Here's how the part is built. I have some questions about the finished solid (model axes, mm). Face numbers are marked on the shaded views. Give positions to 0.01 mm unless a question says otherwise; leave off trailing zeros. Loops run counter-clockwise (first coordinate to the right, second up) from the corner with the lowest first, then second, coordinate; pieces in that order, holes last. Notation, with made-up numbers: (-14, 63) - (-5, 63) arc R20 ccw to (-5, 93) - close; hole circle Ø10 at (64, 58). An arc over 180 degrees is marked (long way). Use one line per item in the form item = value.
Autodesk Inventor part; units mm, degrees
ref_plane "YZ Plane" through (0, 0, 0) normal (1, 0, 0) x (0, 1, 0)
ref_plane "XZ Plane" through (0, 0, 0) normal (0, 1, 0) x (-1, 0, 0)
ref_plane "XY Plane" through (0, 0, 0) normal (0, 0, 1) x (1, 0, 0)
sketch "Sketch1" plane through (0, 0, 0) normal (0, 0, 1) x (1, 0, 0)
  line L0 (0, 31.75) -> (12.7, 31.75)
  line L1 (12.7, 31.75) -> (12.7, -31.75)
  line L2 (12.7, -31.75) -> (0, -31.75)
  line L3 (0, -31.75) -> (0, 31.75)
  point P0 (0, 0)
  point P1 (0, 0)
  dimension "d0" = 25.4
  dimension "d1" = 63.5
revolve "Revolution1" add sketch "Sketch1" angle 360 about axis through (0, -31.75, 0) along (0, 1, 0)
sketch "Sketch2" plane through (0, 0, 0) normal (0, 0, 1) x (1, 0, 0)
  line L0 (0, -35.56) -> (0, 35.56)
  line L1 (0, 25.4) -> (60.325, 25.4)
  line L2 (60.325, 25.4) -> (60.325, -25.4)
  line L3 (60.325, -25.4) -> (0, -25.4)
  line L4 (0, -25.4) -> (0, 25.4)
  circle A0 centre (60.325, 0) radius 25.4
  point P0 (0, 0)
  dimension "d3" = 60.325
  dimension "d4" = 50.8
extrude "Extrusion1" add sketch "Sketch2" along normal mid plane 25.4
sketch "Sketch3" plane through (0, 31.75, 0) normal (0, 1, 0) x (1, 0, 0)
  circle A0 centre (0, 0) radius 12.7
  circle A1 centre (0, 0) radius 7.9375
  dimension "d7" = 15.875
extrude "Extrusion2" cut sketch "Sketch3" against normal through all contours A1
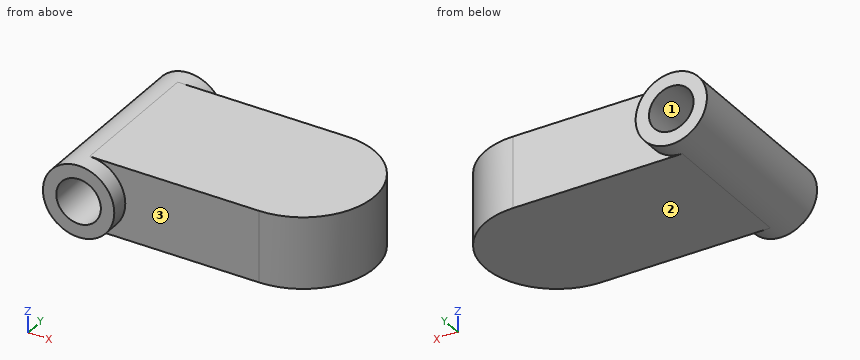
(1) If we section it at B-B (y = 0): List the corners of the cut face in (x, z) for me (1 decimal), plus the area to 3 significant figures.
Geometry says:
outline = (0, -12.7) - (85.7, -12.7) - (85.7, 12.7) - (0, 12.7) arc R12.7 ccw to start; hole circle Ø15.9 at (0, 0)
area = 2,230 mm²
(2) If we section it at D-D (x = 57.5): List the corners of the cut face in (y, z) for me.
Geometry says:
outline = (-25.4, -12.7) - (25.4, -12.7) - (25.4, 12.7) - (-25.4, 12.7) - close
(3) If I drill on probe 1 along Z at (x, y) = (0, -17); probe 2 along X at (y, z) = (12.5, -5); probe 3 along X at (y, z) = (14, 0), over which ranges is the centre line in solid material (lowest first)?
Geometry says:
probe_1 = -12.7 to -7.94, 7.94 to 12.7
probe_2 = -11.67 to -6.16, 6.16 to 82.44
probe_3 = -12.7 to -7.94, 7.94 to 81.52
(4) If we section it at C-C (x = -3): List the corners of the cut face in (y, z) for me.
Geometry says:
outline = (-31.75, -12.34) - (31.75, -12.34) - (31.75, -7.35) - (-31.75, -7.35) - close; (-31.75, 7.35) - (31.75, 7.35) - (31.75, 12.34) - (-31.75, 12.34) - close
(5) For P1, Ø12.5, axis at x = 39, z = -3, coming from the +Y side; P2, Ø5, axis at y = -5, z = 9, coming from the +X side; P3, Ø2, axis at y = -11.5, z = 5.5, coming from the -X side, each with a flat end and sliding along its axis, tell me the tip position at first contact or that it passes through.
Geometry says:
P1 = 25.4
P2 = 85.6
P3 = -11.88
(6) Thinking about a two-plate mould opening in Z: for the marked faces 1, 2 and 3, which applies, pulls with the +Z half, pulls with the -Z half, needs draft (parallel to the pull), parting line crosses it, or undercut?
Geometry says:
face_1 = undercut
face_2 = pulls with the -Z half
face_3 = needs draft
